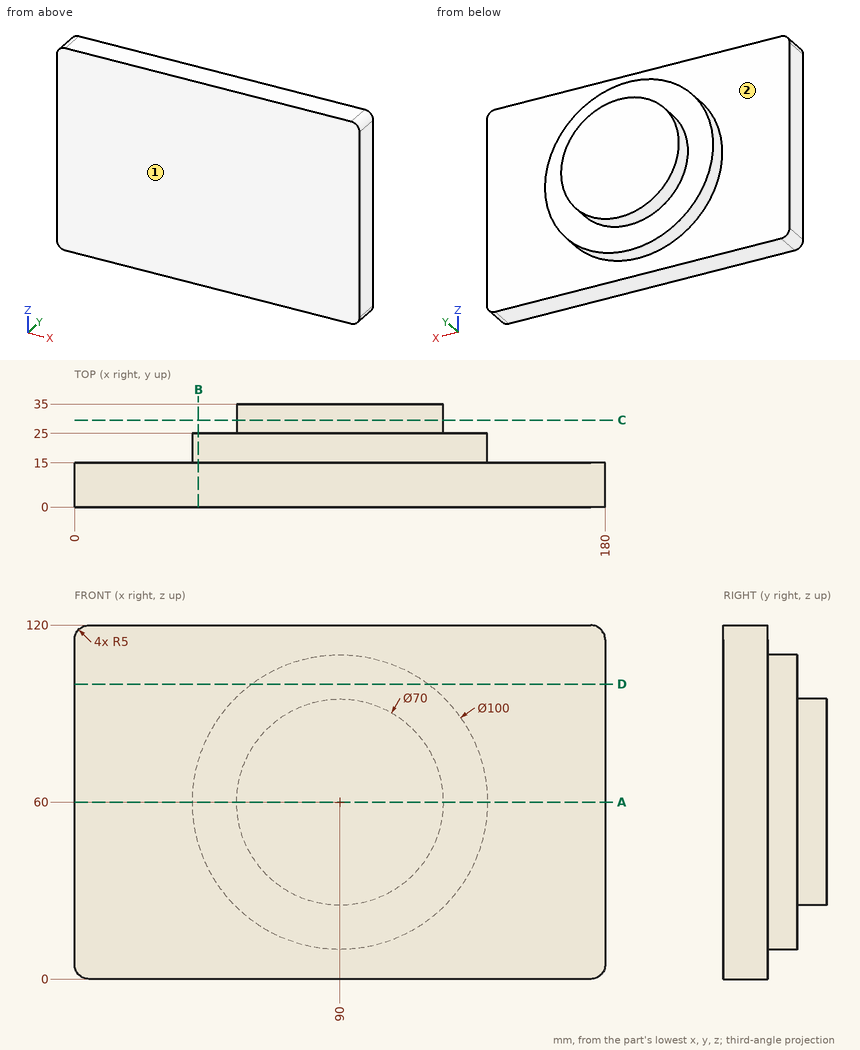
Can you work these out from the drawing? Everything is in mm from the part's minimum corner. A direction names the side the tool comes from. Give positions to 0.01 mm unless a question says otherwise; leave off trailing zeros. Order: outer loops, then holes, each group sorted by start corner. A loop starts at its lowest first (then second) coordinate and runs counter-clockwise, first axis right, second up.
Item 1: If we section it at B-B, the plane x = 42: Write out the boundary of the cut face in (y, z), plus the area to 3 significant figures.
Item 2: If we section it at D-D, the plane z = 100: Write out the boundary of the cut face in (x, y).
Item 3: If we section it at C-C, the plane y = 29.5: Write out the boundary of the cut face in (x, z).
Item 4: For the marked faces 1 and 2, which set-ups out of +Z, -Z, +X, -X, +Y, -Y let a thin tool reach every point of the face, with its end or its side?
Item 5: If we section it at A-A, the plane z = 60: Write out the boundary of the cut face in (x, y), plus the area to 3 significant figures.
Item 6: I need wall thicknesses on line 1 (Y direction, x = 156, z = 22.5); line 2 (Y direction, x = 71, z = 92); line 3 (Z direction, x = 85, y = 28.5). Which ranges of each line are inside material? Lowest first, please.
Item 7: I'm going to push flat-ended pins straight in: pin 1 (8 mm diameter, centred on x = 93, y = 28.5, fed in from +Z); pin 2 (1.5 mm diameter, centred on x = 53, y = 28, fed in from -Z); pin 3 (12 mm diameter, centred on x = 101.5, y = 24.5, fed in from -Z); pin 4 (8 mm diameter, centred on x = 118, z = 17, fed in from +Y). Where does each tip first touch, or does it pass through?
Values:
1. outline: (0, 0) - (15, 0) - (15, 46) - (25, 46) - (25, 74) - (15, 74) - (15, 120) - (0, 120) - close
1. area: 2,080 mm2
2. outline: (0, 0) - (180, 0) - (180, 15) - (120, 15) - (120, 25) - (60, 25) - (60, 15) - (0, 15) - close
3. outline: circle Ø70 at (90, 60)
4. face 1: +Z, -Z, +X, -X, -Y
4. face 2: +Y
5. outline: (0, 0) - (180, 0) - (180, 15) - (140, 15) - (140, 25) - (125, 25) - (125, 35) - (55, 35) - (55, 25) - (40, 25) - (40, 15) - (0, 15) - close
5. area: 4,400 mm2
6. line 1: y = 0 to 15
6. line 2: y = 0 to 25
6. line 3: z = 25.36 to 94.64
7. pin 1: stops at z = 109.99
7. pin 2: passes through
7. pin 3: stops at z = 10.3
7. pin 4: stops at y = 25
